```python
from build123d import *

# Parameters (mm, degrees)
SKETCH3_R         = 7.14375
GEARBODY_DEPTH    = 6.35
TOOTHCUT_DEPTH    = 12.932679
CIRPATTERN1_COUNT = 16
HUB1DIA_R         = 4.7625
HUB1_DEPTH        = 5.080000076
BOREDIA_R         = 2.514599986
BORE_DEPTH        = 12700
SS1HUB1_D         = 2.27584
SS1HUB1_DEPTH     = 4.7625
SS1HUB1_TIP       = 0.683731316


with BuildPart() as part:
    # Sketch3 → gearBody (new body)
    with BuildSketch(Plane.XY):
        Circle(SKETCH3_R)
    extrude(amount=GEARBODY_DEPTH)

    # Sketch2 → toothCut (cut, through all)
    with BuildSketch(Plane.XY):
        with BuildLine():
            ThreePointArc((5.306900665, -0.651157603), (5.318245312, -0.550879014), (5.327695278, -0.450404168))
            ThreePointArc((5.327695278, -0.450404168), (5.423940856, -0.248073769), (5.629653426, -0.159286719))
            ThreePointArc((5.629653426, -0.159286719), (6.706703242, 0.149132804), (7.533202253, 0.905478157))
            ThreePointArc((7.533202253, 0.905478157), (7.547045935, -0.781744537), (7.187671981, -2.430308285))
            ThreePointArc((7.187671981, -2.430308285), (6.533745871, -1.520616276), (5.542778599, -0.997985647))
            ThreePointArc((5.542778599, -0.997985647), (5.359631891, -0.868919444), (5.306900665, -0.651157603))
        make_face()
    toothcut = extrude(amount=TOOTHCUT_DEPTH, mode=Mode.SUBTRACT)

    # CirPattern1: toothCut ×16 about axis
    cirpattern1_axis = Axis((0, 0, 0), (0, 0, 1))
    for i in range(1, CIRPATTERN1_COUNT):
        add(toothcut.rotate(cirpattern1_axis, i * 360 / CIRPATTERN1_COUNT), mode=Mode.SUBTRACT)

    # hub1Dia → hub1 (add)
    with BuildSketch(Plane(origin=(0, 0, 0), x_dir=(-1, 0, 0), z_dir=(0, 0, -1))):
        with Locations(Location((0, 0, 0), (0, 0, 180))):
            Circle(HUB1DIA_R)
    extrude(amount=HUB1_DEPTH)

    # boreDia → bore (cut, symmetric)
    with BuildSketch(Plane.XY):
        Circle(BOREDIA_R)
    extrude(amount=BORE_DEPTH, both=True, mode=Mode.SUBTRACT)

    # ss1Hub1
    with Locations(Plane(origin=(4.188781818, -2.266167057, -2.540000038), x_dir=(0.475835602514, 0.879534240027, 0), z_dir=(0.879534240027, -0.475835602514, 0))):
        with Locations((0, 0)):
            Hole(SS1HUB1_D / 2, depth=SS1HUB1_DEPTH)
            with Locations((0, 0, -(SS1HUB1_DEPTH + SS1HUB1_TIP / 2))):  # 118° drill point
                Cone(0, SS1HUB1_D / 2, SS1HUB1_TIP, mode=Mode.SUBTRACT)


solid = part.part
```
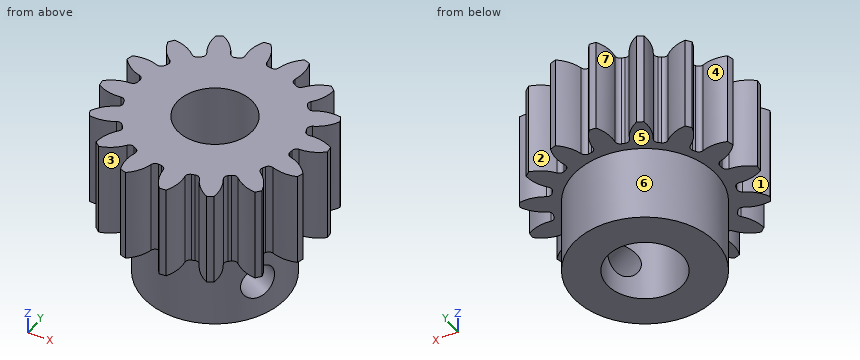
Design review of the part built by this model. Coordinates are the model's own, in mm. Face numbers are marked on the shaded views. A direction names the side the tool comes from. Coordinates: 2 decimals unless noted, no trailing zeros. Order: outer loops, then holes, each group sorted by start corner. A loop starts at its lowest first (then second) coordinate and runs counter-clockwise, first axis right, second up. Notation, with made-up numbers: M 9.25,62 L 49.25,62 A19 ccw 49.25,77 Z; hole C 89,42 d7. An arc over 180 degrees is marked long. Answer as a JSON object with one key per item and string values. Group by question number.
1) Add section B-B, the plane z = -2.25. Write out the cut boundary in (x, y) (1 decimal), then the cut area to 3 significant figures.
2) Mouldability with a two-part tool opening along Y and no side actions: class the marked faces 5, 6 and 7 as pulls with the +Y half, pulls with the -Y half, needs draft (parallel to the pull), parting line crosses it, or undercut.
3) Wall thickness on L1, parallel to Y at x = -1, z = -3; L2, parallel to Y at x = 6.25, z = 4; L3, parallel to Z at x = 4.5, y = 2: over which ranges is each line inside the solid? List them lowest first.
4) Add section A-A, the plane z = -4.5. Write out the cut boundary in (x, y) (1 decimal), then the cut area to 3 significant figures.
5) For pin 1 (1.5 mm diameter, centred on y = -2.5, z = 2, fed in from +X); pin 2 (3 mm diameter, centred on x = 4, y = 5.5, fed in from -Z); pin 3 (3 mm diameter, centred on x = 1.5, z = -3.5, fed in from +Y), all flat-tipped, find the tip position at first contact; note any pin that passes through.
6) Tool access review of the marked faces 1, 2, 3 and 4: name each direction out of +Z, -Z, +X, -X, +Y, -Y from which nothing blocks a thin tool from reaching the whole face with its end or side.
Computed values:
{
 "1": {"outline": "M 1.5,-2 A2.5 cw long 2.5,-0.1 L 4.6,-1.2 A4.8 ccw long 3.6,-3.2 Z", "area": "46.4 mm^2"},
 "2": {"face 5": "needs draft", "face 6": "parting line crosses it", "face 7": "undercut"},
 "3": {"L1": "y = -4.66 to -2.31, 2.31 to 4.66", "L2": "y = -2.43 to -1.31, -0.05 to 1.19, 2.86 to 3.46", "L3": "z = 0 to 6.35"},
 "4": {"outline": "C 0,0 d9.5; hole C 0,0 d5", "area": "51.4 mm^2"},
 "5": {"pin 1": "stops at x = 6.89", "pin 2": "stops at z = 0", "pin 3": "stops at y = 4.76"},
 "6": {"face 1": "+Z, -Z, -X", "face 2": "+Z, -Z, +Y", "face 3": "+Z, -Z, -Y", "face 4": "+Z, -Z"}
}
